Answer from the drawing. Dimensions are ordinates in mm from the lowest x, y and z of the part. Round coordinates to 2 decimals unless told otherwise and drop trailing zeros. Order: outer loops, then holes, each group sorted by start corner. A loop starts at its lowest first (then second) coordinate and runs counter-clockwise, first axis right, second up. Notation, with made-up numbers: (-15.75, 21.5) -> (7.25, 21.5) arc R21 cw to (7.25, 49.5) -> close; hole circle Ø5 at (82.25, 80). An arc over 180 degrees is marked (long way). Use a Markdown table: item, result. Add a question column.
1. Section C-C, the plane z = 61 is taken. Give the vertices of the cut face in (x, y), then the cut area to 3 significant figures.
2. Consider L1, parallel to Z at x = 146.05, y = 4.5; L2, parallel to X at y = 2, z = 38.1; L3, parallel to Z at x = 46, y = 5.5. Determine where each line is inside the solid, lowest interval first. Write a range as [from, to].
3. Section B-B, the plane z = 38.1 is taken. Give the vertices of the cut face in (x, y), then the cut area to 3 significant figures.
4. Section A-A, the plane x = 146.05 is taken. Give the vertices of the cut face in (y, z), then the cut area to 3 significant figures.
5. Given pin 1 (1 mm diameter, centred on y = 5, z = 17, fed in from +X); pin 2 (1.9 mm diameter, centred on x = 53, y = 4.5, fed in from +Z); pin 3 (2 mm diameter, centred on x = 231, y = 4.5, fed in from -Z), each flat-ended and moving along its own axis, determine where each tip first touches the part or whether it passes through.
6. Section D-D, the plane x = 257 is taken. Give the vertices of the cut face in (y, z), then the cut area to 3 significant figures.
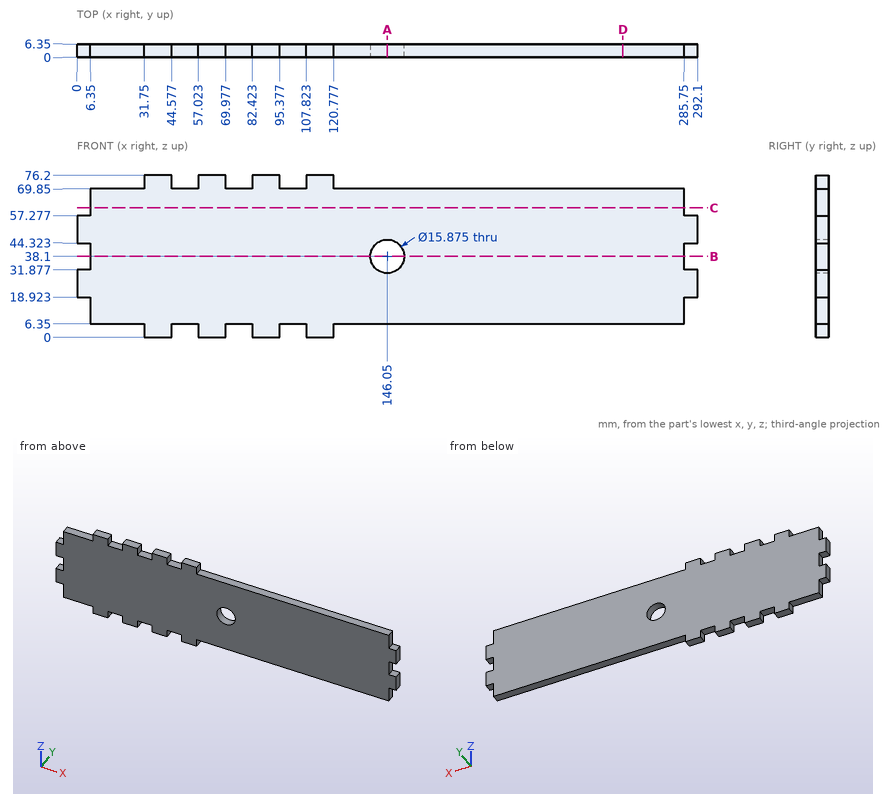
Verdict:
| question | item | result |
|---|---|---|
| 1 | outline | (6.35, 0) -> (285.75, 0) -> (285.75, 6.35) -> (6.35, 6.35) -> close |
| 1 | area | 1,770 mm2 |
| 2 | L1 | z = [6.35, 30.16], [46.04, 69.85] |
| 2 | L2 | x = [6.35, 138.11], [153.99, 285.75] |
| 2 | L3 | z = [6.35, 69.85] |
| 3 | outline | (6.35, 0) -> (138.11, 0) -> (138.11, 6.35) -> (6.35, 6.35) -> close; (153.99, 0) -> (285.75, 0) -> (285.75, 6.35) -> (153.99, 6.35) -> close |
| 3 | area | 1,670 mm2 |
| 4 | outline | (0, 6.35) -> (6.35, 6.35) -> (6.35, 30.16) -> (0, 30.16) -> close; (0, 46.04) -> (6.35, 46.04) -> (6.35, 69.85) -> (0, 69.85) -> close |
| 4 | area | 302 mm2 |
| 5 | pin 1 | stops at x = 285.75 |
| 5 | pin 2 | stops at z = 69.85 |
| 5 | pin 3 | stops at z = 6.35 |
| 6 | outline | (0, 6.35) -> (6.35, 6.35) -> (6.35, 69.85) -> (0, 69.85) -> close |
| 6 | area | 403 mm2 |
